The drawing under review shows one solid part. Ordinate dimensions are in mm from its lowest x, y, z. A direction names the side the tool comes from. Coordinates: 2 decimals unless noted, no trailing zeros. Loops run counter-clockwise (first coordinate to the right, second up) from the corner with the lowest first, then second, coordinate; pieces in that order, holes last. Notation, with made-up numbers: (81, 12) - (116, 12) arc R9 cw to (116, 21) - close; hole circle Ø1 at (23.25, 47). An arc over 180 degrees is marked (long way). Answer as a JSON object with one key per item and string values. Group by question number.
Item 1: Clearance check with flat-ended pins moving along their axes: pin 1 (4 mm diameter, centred on x = 5.5, y = 5.5, fed in from +Z); pin 2 (6 mm diameter, centred on x = 2.5, y = 3, fed in from -Z); pin 3 (2 mm diameter, centred on y = 9.5, z = 22, fed in from -X); pin 4 (1 mm diameter, centred on x = 8.5, z = 27.5, fed in from -Y). State where each tip first meets the part, or that it passes through.
Item 2: We need section A-A (z = 39). Give the boundary of the cut face in (x, y), then the cut area to 3 significant figures.
Item 3: We need section B-B (z = 26.5). Give the boundary of the cut face in (x, y).
Item 4: To check wall thickness, follow line 1 (Y direction, x = 5.5, z = 5); line 2 (X direction, y = 3.5, z = 45.5); line 3 (X direction, y = 4.5, z = 43). State the ranges of each line that lie inside material, in increasing order.
Item 5: Tool access review of the marked faces 1, 2 and 3: name each direction out of +Z, -Z, +X, -X, +Y, -Y from which nothing blocks a thin tool from reaching the whole face with its end or side.
Item 6: We need section C-C (y = 10.25). Give the boundary of the cut face in (x, z), then the cut area to 3 significant figures.
Item 7: We need section D-D (x = 1.75). Give the boundary of the cut face in (y, z).
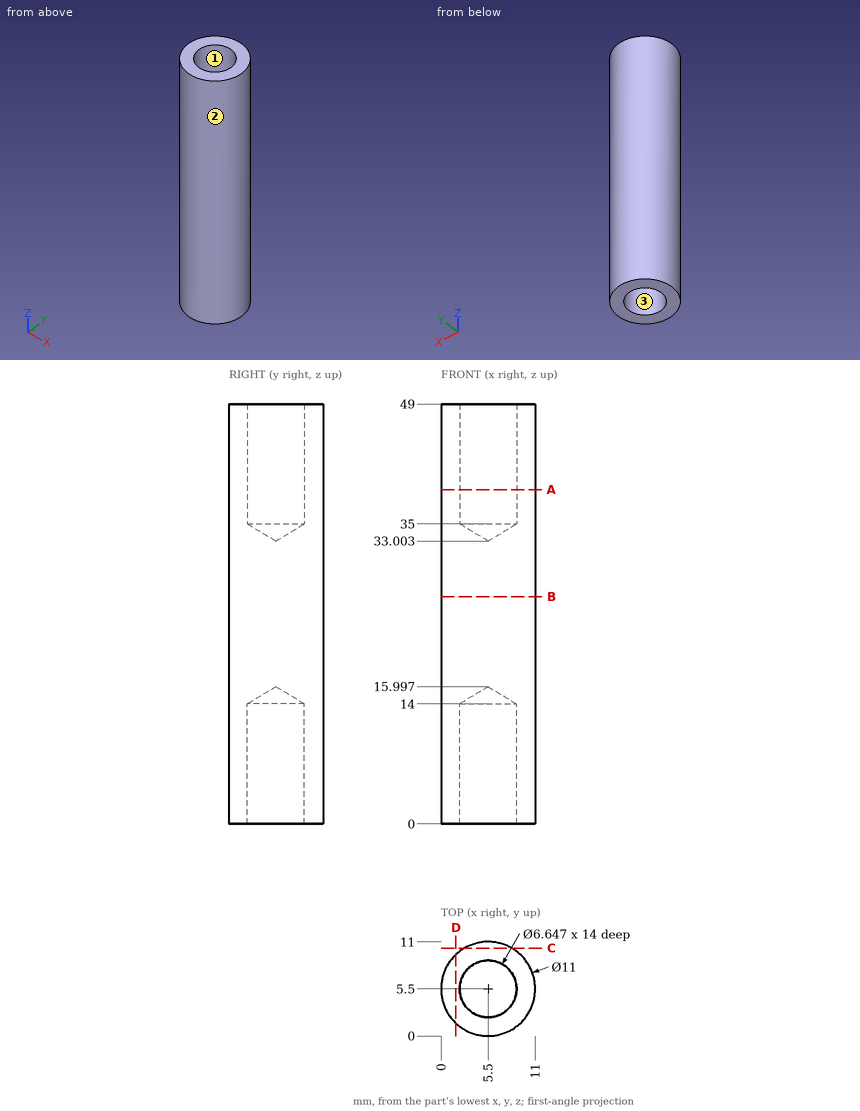
Check sheet entries:
{
 "1": {"pin 1": "stops at z = 34.2", "pin 2": "stops at z = 0", "pin 3": "stops at x = 0.89", "pin 4": "stops at y = 0.6"},
 "2": {"outline": "circle Ø11 at (5.5, 5.5); hole circle Ø6.65 at (5.5, 5.5)", "area": "60.3 mm2"},
 "3": {"outline": "circle Ø11 at (5.5, 5.5)"},
 "4": {"line 1": "y = 0 to 2.18, 8.82 to 11", "line 2": "x = 0.38 to 2.85, 8.15 to 10.62", "line 3": "x = 0.09 to 2.33, 8.67 to 10.91"},
 "5": {"face 1": "+Z", "face 2": "+Z, -Z", "face 3": "-Z"},
 "6": {"outline": "(2.73, 0) - (8.27, 0) - (8.27, 49) - (2.73, 49) - close", "area": "272 mm2"},
 "7": {"outline": "(1.48, 0) - (9.52, 0) - (9.52, 49) - (1.48, 49) - close"}
}
